Here's the drawing with two shaded views (mm, measured from the low corner). I have some questions. A direction names the side the tool comes from. Coordinates: 2 decimals unless noted, no trailing zeros. Write each loop counter-clockwise with the first axis right and the second up, starting at its lowest first coordinate (ties: lowest second). Pieces come first, ordered by that corner, then holes. Notation, with made-up numbers: (-33.5, -37.5) -> (11.5, -37.5) arc R32 cw to (11.5, -9.5) -> close; hole circle Ø4 at (9, 61.25). An arc over 180 degrees is marked (long way). Use a Markdown table: item, result. Add a question column.
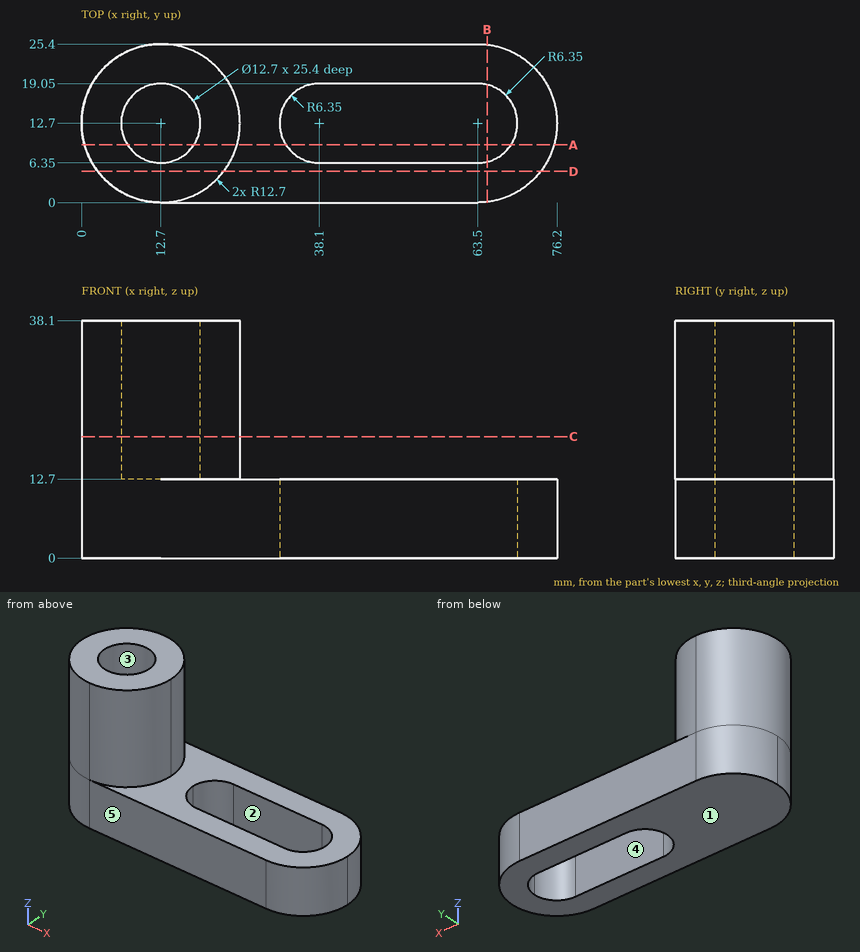
Q1. Please list where these lines run through material, in increasing order: line 1 (Y direction, x = 12.7, z = 22.5); line 2 (Z direction, x = 72.5, y = 8.5).
Q2. Thinking about a two-plate mould opening in X: for the marked faces 4 and 5, which applies, released by +X, released by -X, zero draft, split by the parting line, or undercut?
Q3. Suppose I cut it at A-A, the plane y = 9.25. Write out the boundary of the cut face in (x, z), and give its area (3 significant figures).
Q4. Suppose I cut it at B-B, the plane x = 65. Write out the boundary of the cut face in (y, z).
Q5. Suppose I cut it at D-D, the plane y = 5. Write out the boundary of the cut face in (x, z).
Q6. Which directions (+Z, -Z, +X, -X, +Y, -Y) give clear straight access to the entire face, cutting with the end or side of a thin tool? Please do the marked faces 1, 2 and 3.
Q7. Will these pins go through, and if not, where does the flat tip stop? pin 1 (8 mm diameter, centred on y = 17, z = 33, fed in from -X); pin 2 (1 mm diameter, centred on y = 22.5, z = 21, fed in from +X); pin 3 (1.5 mm diameter, centred on y = 6, z = 21, fed in from -X).
Q8. Suppose I cut it at C-C, the plane z = 19.5. Write out the boundary of the cut face in (x, y).
Answer key:
| question | item | result |
|---|---|---|
| 1 | line 1 | y = 0 to 6.35, 19.05 to 25.4 |
| 1 | line 2 | z = 0 to 12.7 |
| 2 | face 4 | undercut |
| 2 | face 5 | zero draft |
| 3 | outline | (0.48, 0) -> (32.77, 0) -> (32.77, 12.7) -> (24.92, 12.7) -> (24.92, 38.1) -> (18.03, 38.1) -> (18.03, 12.7) -> (7.37, 12.7) -> (7.37, 38.1) -> (0.48, 38.1) -> close; (68.83, 0) -> (75.72, 0) -> (75.72, 12.7) -> (68.83, 12.7) -> close |
| 3 | area | 848 mm^2 |
| 4 | outline | (0.09, 0) -> (6.53, 0) -> (6.53, 12.7) -> (0.09, 12.7) -> close; (18.87, 0) -> (25.31, 0) -> (25.31, 12.7) -> (18.87, 12.7) -> close |
| 5 | outline | (2.6, 0) -> (73.6, 0) -> (73.6, 12.7) -> (22.8, 12.7) -> (22.8, 38.1) -> (2.6, 38.1) -> close |
| 6 | face 1 | -Z, +X, -X, +Y, -Y |
| 6 | face 2 | +Z, -Z |
| 6 | face 3 | +Z |
| 7 | pin 1 | stops at x = 0 |
| 7 | pin 2 | stops at x = 21.35 |
| 7 | pin 3 | stops at x = 1.48 |
| 8 | outline | circle Ø25.4 at (12.7, 12.7); hole circle Ø12.7 at (12.7, 12.7) |
